from build123d import *

# Parameters (mm, degrees)
F1_DEPTH = 13.5
F3_DEPTH = 1.2
F5_DEPTH = 1.8


with BuildPart() as f1:
    # F0 (on Top) → F1 (new body)
    with BuildSketch(Plane.XY):
        with BuildLine():
            Line((-8.6, 0), (-8.6, -2.5))
            Line((-8.6, -2.5), (-7, -2.5))
            Line((-7, -2.5), (-7, 0))
            ThreePointArc((-7, 0), (-6.12132, 2.12132), (-4, 3))
            Line((-4, 3), (-0.8, 3))
            Line((-0.8, 3), (-0.8, 1.83303))
            ThreePointArc((-0.8, 1.83303), (0, -2), (0.8, 1.83303))
            Line((0.8, 1.83303), (0.8, 3))
            Line((0.8, 3), (4, 3))
            ThreePointArc((4, 3), (6.12132, 2.12132), (7, 0))
            Line((7, 0), (7, -2.5))
            Line((7, -2.5), (8.6, -2.5))
            Line((8.6, -2.5), (8.6, 0))
            ThreePointArc((8.6, 0), (7.252691, 3.252691), (4, 4.6))
            Line((4, 4.6), (-4, 4.6))
            ThreePointArc((-4, 4.6), (-7.252691, 3.252691), (-8.6, 0))
        make_face()
    extrude(amount=F1_DEPTH)

    # F2 (on face) → F3 (join)
    with BuildSketch(Plane(origin=(0, 0, 0), x_dir=(1, 0, 0), z_dir=(0, 0, -1))):
        with BuildLine():
            Line((-7, 2.5), (-8.6, 2.5))
            Line((-8.6, 2.5), (-8.6, 0))
            ThreePointArc((-8.6, 0), (-7.252691, -3.252691), (-4, -4.6))
            Line((-4, -4.6), (4, -4.6))
            ThreePointArc((4, -4.6), (7.252691, -3.252691), (8.6, 0))
            Line((8.6, 0), (8.6, 2.5))
            Line((8.6, 2.5), (7, 2.5))
            Line((7, 2.5), (7, 3.7))
            Line((7, 3.7), (-7, 3.7))
            Line((-7, 3.7), (-7, 2.5))
        make_face()
    extrude(amount=-F3_DEPTH)

    # F4 (on face) → F5 (join)
    with BuildSketch(Plane.XY.offset(1.2)):
        with BuildLine():
            Line((-3.5, 3), (-3.5, 0))
            ThreePointArc((-3.5, 0), (0, -3.5), (3.5, 0))
            Line((3.5, 0), (3.5, 3))
            Line((3.5, 3), (-3.5, 3))
        make_face()
    extrude(amount=F5_DEPTH)


solid = f1.part
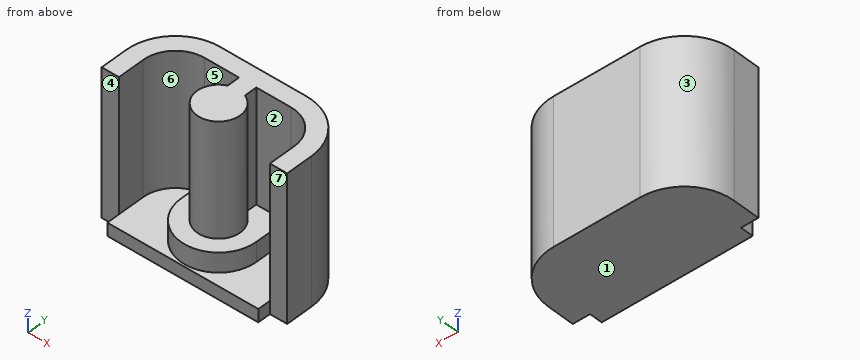
Could you check a few things on this model? Use its own coordinates, in mm. Face numbers are marked on the shaded views. A direction names the side the tool comes from. Give positions to 0.01 mm unless a question says otherwise; leave off trailing zeros. Order: outer loops, then holes, each group sorted by start corner. A loop starts at its lowest first (then second) coordinate and runs counter-clockwise, first axis right, second up. Notation, with made-up numbers: (-6.75, -26) - (0.25, -26) arc R26 ccw to (0.25, -9) - close; hole circle Ø5 at (11, 6). An arc over 180 degrees is marked (long way). One line per question, with ' | ' between items. Start each with the question number.
Item 1: I want a section at C-C on y = -1. Write out the boundary of the cut face in (x, z).
Item 2: I'm going to push flat-ended pins straight in: pin 1 Ø1.5 at (y, z) = (1, 6.5) entering from -X; pin 2 Ø1.3 at (y, z) = (2, 6) entering from -X; pin 3 Ø4 at (x, y) = (-4.5, -1) entering from +Z. Where does each tip first touch, or does it pass through?
Item 3: I want a section at A-A on z = 5.25. Write out the boundary of the cut face in (x, y), then the cut area to 3 significant figures.
Item 4: I need wall thicknesses on probe 1 along X at (y, z) = (-0.5, 12.5); probe 2 along X at (y, z) = (-1, 8.5); probe 3 along Z at (x, y) = (-6.5, -1.5). Which ranges of each line are inside material? Lowest first, please. Write a range as [from, to].
Item 5: I want a section at D-D on x = 1.75. Write out the boundary of the cut face in (y, z).
Item 6: For the marked faces 4, 5, 6 and 7, which set-ups out of +Z, -Z, +X, -X, +Y, -Y let a thin tool reach every point of the face, with its end or its side?
Item 7: Thinking about a two-plate mould opening in Y: for the marked faces 1, 2 and 3, which applies, pulls with the +Y half, pulls with the -Y half, needs draft (parallel to the pull), parting line crosses it, or undercut?
Item 8: I want a section at B-B on x = 0. Write out the boundary of the cut face in (y, z).
Verdict:
1) outline: (-8.6, 0) - (8.6, 0) - (8.6, 13.5) - (7, 13.5) - (7, 1.2) - (3.35, 1.2) - (3.35, 3) - (1.73, 3) - (1.73, 13.5) - (-1.73, 13.5) - (-1.73, 3) - (-3.35, 3) - (-3.35, 1.2) - (-7, 1.2) - (-7, 13.5) - (-8.6, 13.5) - close
2) pin 1: x = -8.59 | pin 2: x = -8.4 | pin 3: z = 3
3) outline: (-8.6, -2.5) - (-7, -2.5) - (-7, 0) arc R3 cw to (-4, 3) - (-0.8, 3) - (-0.8, 1.83) arc R2 ccw (long way) to (0.8, 1.83) - (0.8, 3) - (4, 3) arc R3 cw to (7, 0) - (7, -2.5) - (8.6, -2.5) - (8.6, 0) arc R4.6 ccw to (4, 4.6) - (-4, 4.6) arc R4.6 ccw to (-8.6, 0) - close | area: 54.2 mm^2
4) probe 1: [-8.6, -7], [-1.94, 1.94], [7, 8.6] | probe 2: [-8.6, -7], [-1.73, 1.73], [7, 8.6] | probe 3: [0, 1.2]
5) outline: (-3.7, 0) - (4.6, 0) - (4.6, 13.5) - (3, 13.5) - (3, 3) - (0.97, 3) - (0.97, 13.5) - (-0.97, 13.5) - (-0.97, 3) - (-3.03, 3) - (-3.03, 1.2) - (-3.7, 1.2) - close
6) face 4: +Z, -Z, -X, -Y | face 5: +Z | face 6: +Z, -Y | face 7: +Z, -Z, +X, -Y
7) face 1: needs draft | face 2: undercut | face 3: pulls with the +Y half
8) outline: (-3.7, 0) - (4.6, 0) - (4.6, 13.5) - (-2, 13.5) - (-2, 3) - (-3.5, 3) - (-3.5, 1.2) - (-3.7, 1.2) - close
